CAD build for the part. Positions are in the model's coordinates, mm. A direction names the side the tool comes from. Give positions to 0.01 mm unless a question says otherwise; leave off trailing zeros. Loops run counter-clockwise (first coordinate to the right, second up) from the corner with the lowest first, then second, coordinate; pieces in that order, holes last.
```python
from build123d import *

# Parameters (mm, degrees)
SKETCH_1_R          = 11.5
SKETCH_1_R_2        = 1
SKETCH_1_R_3        = 5
EXTRUDE_1_DEPTH     = 2
SKETCH_1_3_R        = 5
EXTRUDE_2_DEPTH     = 0.25
SKETCH_2_R          = 14
EXTRUDE_3_DEPTH     = 12
EXTRUDE_START       = 1
SKETCH_3_R          = 5
EXTRUDE_4_DEPTH     = 1
CUT_EXTRUDE_START   = -10
SKETCH_3_3_R        = 1
CUT_EXTRUDE_1_DEPTH = 10
CUT_EXTRUDE_2_DEPTH = 3.5
SKETCH_5_W          = 32
SKETCH_5_H          = 32
SKETCH_5_R          = 1.4
EXTRUDE_5_DEPTH     = 2
EXTRUDE_START_2     = 2
SKETCH_6_R          = 1
EXTRUDE_6_DEPTH     = 2
SKETCH_7_W          = 20
SKETCH_7_H          = 20
SKETCH_7_R          = 1.6
EXTRUDE_7_DEPTH     = 1.7


with BuildPart() as part:
    # Sketch 1 → Extrude 1 (new body)
    # profile 1 of 2: a face of its own
    with BuildSketch(Plane(origin=(0, 0, 0), x_dir=(1, 0, 0), z_dir=(0, 1, 0))):
        with Locations(Location((0, 0, 0), (0, 0, 270))):
            Circle(SKETCH_1_R)
        with Locations(Location((0, 8, 0), (0, 0, 270))):
            Circle(SKETCH_1_R_2, mode=Mode.SUBTRACT)
        with Locations(Location((-8, 0, 0), (0, 0, 270))):
            Circle(SKETCH_1_R_2, mode=Mode.SUBTRACT)
        with Locations(Location((0, -8, 0), (0, 0, 270))):
            Circle(SKETCH_1_R_2, mode=Mode.SUBTRACT)
        with Locations(Location((8, 0, 0), (0, 0, 270))):
            Circle(SKETCH_1_R_2, mode=Mode.SUBTRACT)
        Circle(SKETCH_1_R_3, mode=Mode.SUBTRACT)
    # profile 2 of 2: a face of its own
    with BuildSketch(Plane(origin=(0, 0, 0), x_dir=(1, 0, 0), z_dir=(0, 1, 0))):
        Circle(SKETCH_1_R_3)
    extrude(amount=EXTRUDE_1_DEPTH)

    # Sketch 1_3 → Extrude 2 (add)
    with BuildSketch(Plane(origin=(0, 0, 0), x_dir=(1, 0, 0), z_dir=(0, 1, 0))):
        with Locations(Location((0, 0, 0), (0, 0, 270))):
            Circle(SKETCH_1_3_R)
    extrude(amount=-EXTRUDE_2_DEPTH)

    # Sketch 2 → Extrude 3 (add)
    with BuildSketch(Plane(origin=(0, 2, 0), x_dir=(1, 0, 0), z_dir=(0, 1, 0))):
        with Locations(Location((0, 0, 0), (0, 0, 270))):
            Circle(SKETCH_2_R)
    extrude(amount=EXTRUDE_3_DEPTH)

    # Sketch 3 → Extrude 4 (add)
    with BuildSketch(Plane(origin=(0, 14, 0), x_dir=(1, 0, 0), z_dir=(0, 1, 0)).offset(EXTRUDE_START)):
        with Locations(Location((0, 0, 0), (0, 0, 270))):
            Circle(SKETCH_3_R)
    extrude(amount=-EXTRUDE_4_DEPTH)

    # Sketch 3_3 → Cut-Extrude 1 (cut)
    with BuildSketch(Plane(origin=(0, 14, 0), x_dir=(1, 0, 0), z_dir=(0, 1, 0)).offset(CUT_EXTRUDE_START)):
        with Locations(Location((8, 0, 0), (0, 0, 270))):
            Circle(SKETCH_3_3_R)
        with Locations(Location((0, 8, 0), (0, 0, 270))):
            Circle(SKETCH_3_3_R)
        with Locations(Location((-8, 0, 0), (0, 0, 270))):
            Circle(SKETCH_3_3_R)
        with Locations(Location((0, -8, 0), (0, 0, 270))):
            Circle(SKETCH_3_3_R)
    extrude(amount=CUT_EXTRUDE_1_DEPTH, mode=Mode.SUBTRACT)

    # Sketch 4 → Cut-Extrude 2 (cut)
    with BuildSketch(Plane(origin=(0, 14, 0), x_dir=(1, 0, 0), z_dir=(0, 1, 0))):
        with BuildLine():
            Line((14.495689014, 11.66726189), (8.131727984, 5.303300859))
            ThreePointArc((8.131727984, 5.303300859), (5.303300859, 5.303300859), (5.303300859, 8.131727984))
            Line((5.303300859, 8.131727984), (11.66726189, 14.495689014))
            ThreePointArc((11.66726189, 14.495689014), (14.495689014, 14.495689014), (14.495689014, 11.66726189))
        make_face()
        with BuildLine():
            Line((-11.66726189, -14.495689014), (-5.303300859, -8.131727984))
            ThreePointArc((-5.303300859, -8.131727984), (-5.303300859, -5.303300859), (-8.131727984, -5.303300859))
            Line((-8.131727984, -5.303300859), (-14.495689014, -11.66726189))
            ThreePointArc((-14.495689014, -11.66726189), (-14.495689014, -14.495689014), (-11.66726189, -14.495689014))
        make_face()
    extrude(amount=-CUT_EXTRUDE_2_DEPTH, mode=Mode.SUBTRACT)

    # Sketch 5 → Extrude 5 (add)
    with BuildSketch(Plane.XZ):
        Rectangle(SKETCH_5_W, SKETCH_5_H)
        with Locations(Location((13, 13, 0), (0, 0, 270))):
            Circle(SKETCH_5_R, mode=Mode.SUBTRACT)
        with Locations(Location((-13, 13, 0), (0, 0, 90))):
            Circle(SKETCH_5_R, mode=Mode.SUBTRACT)
        with Locations(Location((13, -13, 0), (0, 0, 90))):
            Circle(SKETCH_5_R, mode=Mode.SUBTRACT)
        with Locations(Location((-13, -13, 0), (0, 0, 270))):
            Circle(SKETCH_5_R, mode=Mode.SUBTRACT)
    extrude(amount=EXTRUDE_5_DEPTH)

    # Sketch 6 → Extrude 6 (add)
    with BuildSketch(Plane.XZ.offset(2).offset(EXTRUDE_START_2)):
        with Locations(Location((8, 0, 0), (0, 0, 90))):
            Circle(SKETCH_6_R)
        with Locations(Location((0, -8, 0), (0, 0, 90))):
            Circle(SKETCH_6_R)
        with Locations(Location((-8, 0, 0), (0, 0, 90))):
            Circle(SKETCH_6_R)
        with Locations(Location((0, 8, 0), (0, 0, 90))):
            Circle(SKETCH_6_R)
    extrude(amount=-EXTRUDE_6_DEPTH)

    # Sketch 7 → Extrude 7 (add)
    with BuildSketch(Plane.XZ.offset(4)):
        Rectangle(SKETCH_7_W, SKETCH_7_H)
        with Locations(Location((7, 7, 0), (0, 0, 270))):
            Circle(SKETCH_7_R, mode=Mode.SUBTRACT)
        with Locations(Location((-7, 7, 0), (0, 0, 90))):
            Circle(SKETCH_7_R, mode=Mode.SUBTRACT)
        with Locations(Location((7, -7, 0), (0, 0, 90))):
            Circle(SKETCH_7_R, mode=Mode.SUBTRACT)
        with Locations(Location((-7, -7, 0), (0, 0, 270))):
            Circle(SKETCH_7_R, mode=Mode.SUBTRACT)
    extrude(amount=EXTRUDE_7_DEPTH)


solid = part.part
```
1. Probe line 1 along Y through (x, z) = (-8, -10.5); line 2 along Y through (x, z) = (9.5, -6); line 3 along X through (y, z) = (4.5, -0.5). List the from-to ranges inside material, lowest first.
Responses:
line 1: y = -2 to 0, 2 to 14
line 2: y = -5.7 to -4, -2 to 14
line 3: x = -13.99 to -8.87, -7.13 to 7.13, 8.87 to 13.99
2. Saw through at D-D, the plane z = 0. Count the separate pieces of the cut face and the enclosed holes in it, and give its area (3 significant figures).
Responses:
separate pieces: 1
enclosed holes: 3
area: 450 mm2
3. Pull direction Z, two halves, no side cores. Call faces 1 (the face through (0, -5.7, 0)), 2 (the face through (9, 9, 0)), 3 (the face through (-12.05, -0.99, -11.97)), 4 (the face through (0, -1, -16)): released by +Z, released by -Z, zero draft, split by the parting line, or undercut.
Responses:
face 1: zero draft
face 2: undercut
face 3: undercut
face 4: released by -Z
4. Saw through at B-B, the plane x = 6.5. List the corners of the cut face in (y, z), and give its area (3 significant figures).
Responses:
outline: (-5.7, -10) - (-4, -10) - (-4, -8.52) - (-5.7, -8.52) - close; (-5.7, -5.48) - (-4, -5.48) - (-4, 5.48) - (-5.7, 5.48) - close; (-5.7, 8.52) - (-4, 8.52) - (-4, 10) - (-5.7, 10) - close; (-2, -16) - (0, -16) - (0, -9.49) - (2, -9.49) - (2, -12.4) - (14, -12.4) - (14, -9.33) - (10.5, -9.33) - (10.5, -4.73) - (14, -4.73) - (14, 12.4) - (2, 12.4) - (2, 9.49) - (0, 9.49) - (0, 16) - (-2, 16) - close
area: 407 mm2
5. Tool access for faces 5 (the face through (0, -1, 16)), 6 (the face through (0, 2, 8)), 7 (the face through (8, 10.5, -8)), 8 (the face through (0, -5, 10)): list every direction of +Z, -Z, +X, -X, +Y, -Y with a clear straight run to the whole face (end or side of a thin tool).
Responses:
face 5: +Z, +X, -X, +Y, -Y
face 6: none
face 7: +Y
face 8: +Z, +X, -X, -Y
6. Saw through at A-A, the plane y = -1. List the corners of the cut face in (x, z), and give its area (3 significant figures).
Responses:
outline: (-16, -16) - (16, -16) - (16, 16) - (-16, 16) - close; hole circle Ø2.8 at (-13, -13); hole circle Ø2.8 at (-13, 13); hole circle Ø2.8 at (13, -13); hole circle Ø2.8 at (13, 13)
area: 999 mm2
7. Saw through at C-C, the plane z = 13. List the corners of the cut face in (x, y), and give its area (3 significant figures).
Responses:
outline: (-16, -2) - (-14.4, -2) - (-14.4, 0) - (-16, 0) - close; (-11.6, -2) - (11.6, -2) - (11.6, 0) - (-11.6, 0) - close; (-5.2, 2) - (5.2, 2) - (5.2, 14) - (-5.2, 14) - close; (14.4, -2) - (16, -2) - (16, 0) - (14.4, 0) - close
area: 178 mm2
8. Drop flat-ended pins along their axis: pin 1 (1 mm diameter, centred on x = 8, z = 0, fed in from +Y); pin 2 (2 mm diameter, centred on x = -6.5, y = 12.5, fed in from -Z); pin 3 (10 mm diameter, centred on y = 8, z = -4.5, fed in from -X); pin 4 (2 mm diameter, centred on x = 13, z = 13, fed in from +Y). Give the stop position or say it passes through.
Responses:
pin 1: stops at y = 4
pin 2: stops at z = -12.87
pin 3: stops at x = -14
pin 4: passes through
